Geometry: final body of the model. Coordinates: model frame, mm. Face numbers are marked on the shaded views. A direction names the side the tool comes from. Give positions to 0.01 mm unless a question says otherwise; leave off trailing zeros. Write each loop counter-clockwise with the first axis right and the second up, starting at its lowest first coordinate (ties: lowest second). Pieces come first, ordered by that corner, then holes.
Q1. Section B-B (y = 2). Return the cut outline in (x, z).
Q2. Pin query (flat end, axial travel): pin 1 Ø4.5 at (y, z) = (-2.09, -13.5) entering from -X; pin 2 Ø4 at (x, y) = (6.5, 1.5) entering from +Z. Return the tip coordinate at first contact, or that it passes through.
Q3. Mould query, pull axis Y, two halves, no side actions, for the marked faces 3, 4, 5 and 6. Classes: +Y half, -Y half, draft (parallel to the pull), parting line (faces both ways), or undercut.
Q4. Section A-A (z = -6.5). Return the cut outline in (x, y), plus the area to 3 significant figures.
Q5. Reachability of the marked faces 1 and 2 from +Z, -Z, +X, -X, +Y, -Y: full face, straight path, thin tool, end or side. Return the list, or none.
Q6. Line query: line 1 (Y direction, x = -9, z = -21); line 2 (X direction, y = -7, z = -15.25); line 3 (Z direction, x = -6.75, y = -8). Output: solid intervals per line, ascending.
Q7. Section C-C (z = -13.5). Return the cut outline in (x, y), plus the area to 3 significant figures.
Q8. Section D-D (x = 0). Return the cut outline in (y, z), plus the area to 3 significant figures.
from build123d import *

# Parameters (mm, degrees)
SKETCH1_W           = 24
SKETCH1_H           = 14
BOSS_EXTRUDE4_DEPTH = 28
SKETCH3_W           = 22
SKETCH3_H           = 12
CUT_EXTRUDE1_DEPTH  = 27
SKETCH4_R           = 6
SKETCH4_R_2         = 2.487873036
CUT_EXTRUDE7_DEPTH  = 5


with BuildPart() as part:
    # Sketch1 → Boss-Extrude4 (new body)
    with BuildSketch(Plane.XY):
        with Locations((2.418604651, -2.093023256)):
            Rectangle(SKETCH1_W, SKETCH1_H)
    extrude(amount=-BOSS_EXTRUDE4_DEPTH)

    # Sketch3 → Cut-Extrude1 (cut)
    with BuildSketch(Plane.XY):
        with Locations((2.418604651, -2.093023256)):
            Rectangle(SKETCH3_W, SKETCH3_H)
    extrude(amount=-CUT_EXTRUDE1_DEPTH, mode=Mode.SUBTRACT)

    # Sketch4 → Cut-Extrude7 (cut)
    with BuildSketch(Plane.ZY.offset(9.581395349)):
        with Locations((-21, -2.093023256)):
            Circle(SKETCH4_R)
        with Locations((-13.5, -2.093023256)):
            Circle(SKETCH4_R_2)
    extrude(amount=-CUT_EXTRUDE7_DEPTH, mode=Mode.SUBTRACT)


solid = part.part
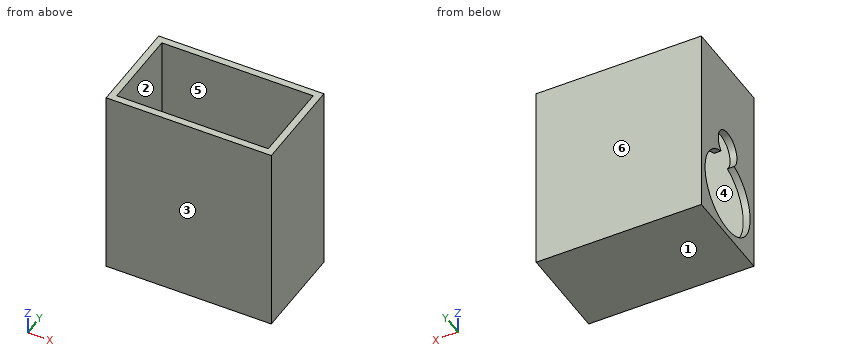
Computed:
1. outline: (-9.58, -28) - (14.42, -28) - (14.42, 0) - (13.42, 0) - (13.42, -27) - (-8.58, -27) - (-8.58, -25.39) - (-9.58, -25.39) - close; (-9.58, -16.61) - (-8.58, -16.61) - (-8.58, 0) - (-9.58, 0) - close
2. pin 1: stops at x = 13.42
2. pin 2: stops at z = -27
3. face 3: -Y half
3. face 4: undercut
3. face 5: undercut
3. face 6: +Y half
4. outline: (-9.58, -9.09) - (14.42, -9.09) - (14.42, 4.91) - (-9.58, 4.91) - close; hole (-8.58, -8.09) - (13.42, -8.09) - (13.42, 3.91) - (-8.58, 3.91) - close
4. area: 72.0 mm2
5. face 1: -Z, +X, -X, +Y, -Y
5. face 2: +Z
6. line 1: y = -9.09 to -8.09, 3.91 to 4.91
6. line 2: x = -9.58 to -8.58, 13.42 to 14.42
6. line 3: z = -28 to -27
7. outline: (-9.58, -9.09) - (14.42, -9.09) - (14.42, 4.91) - (-9.58, 4.91) - (-9.58, 0.39) - (-8.58, 0.39) - (-8.58, 3.91) - (13.42, 3.91) - (13.42, -8.09) - (-8.58, -8.09) - (-8.58, -4.58) - (-9.58, -4.58) - close
7. area: 67.0 mm2
8. outline: (-9.09, -28) - (4.91, -28) - (4.91, 0) - (3.91, 0) - (3.91, -27) - (-8.09, -27) - (-8.09, 0) - (-9.09, 0) - close
8. area: 68.0 mm2
